The drawing under review shows one solid part. Ordinate dimensions are in mm from its lowest x, y, z. A direction names the side the tool comes from. Coordinates: 2 decimals unless noted, no trailing zeros. Loops run counter-clockwise (first coordinate to the right, second up) from the corner with the lowest first, then second, coordinate; pieces in that order, holes last. Notation, with made-up numbers: (11.25, 32) -> (50.25, 32) arc R21 ccw to (50.25, 61) -> close; hole circle Ø9 at (89, 65.5). An arc over 180 degrees is marked (long way). Use a Markdown table: item, result.
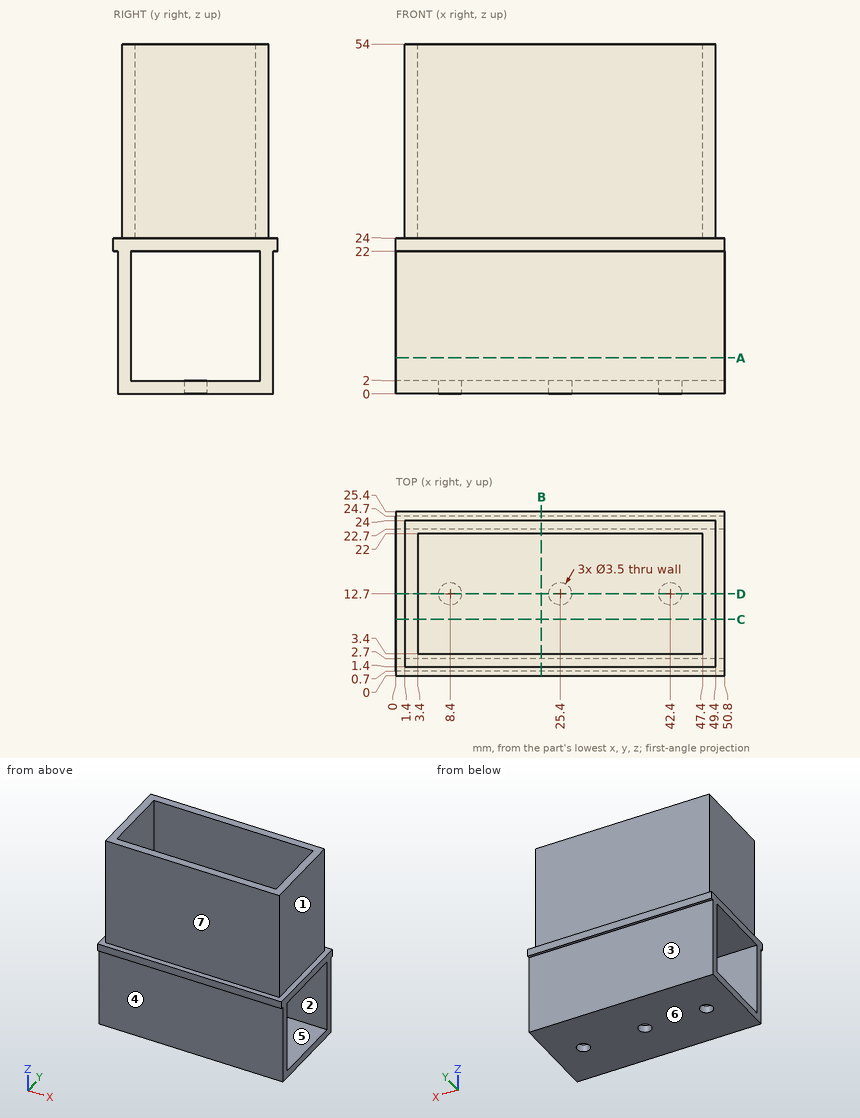
(1) For the marked faces 1, 2, 3 and 4, list the 3-axis set-ups (+Z, -Z, +X, -X, +Y, -Y) from which the entire face can be reached by the end or side of a thin tool; tool diameter is ignored.
Found:
| item | result |
|---|---|
| face 1 | +Z, +X, +Y, -Y |
| face 2 | +X, -X |
| face 3 | -Z, +X, -X, +Y |
| face 4 | -Z, +X, -X, -Y |
(2) Take a section at D-D on y = 12.7. Write out the cut boundary in (x, z), plus the area to 3 significant figures.
Found:
| item | result |
|---|---|
| outline | (0, 0) -> (6.65, 0) -> (6.65, 2) -> (0, 2) -> close; (0, 22) -> (50.8, 22) -> (50.8, 24) -> (49.4, 24) -> (49.4, 54) -> (47.4, 54) -> (47.4, 24) -> (3.4, 24) -> (3.4, 54) -> (1.4, 54) -> (1.4, 24) -> (0, 24) -> close; (10.15, 0) -> (23.65, 0) -> (23.65, 2) -> (10.15, 2) -> close; (27.15, 0) -> (40.65, 0) -> (40.65, 2) -> (27.15, 2) -> close; (44.15, 0) -> (50.8, 0) -> (50.8, 2) -> (44.15, 2) -> close |
| area | 302 mm^2 |
(3) For pin 1 Ø8 at (x, y) = (33.5, 14.5) entering from +Z; pin 2 Ø22 at (x, z) = (32, 7.5) entering from -Y; pin 3 Ø2 at (x, y) = (40, 8) entering from -Z; pin 4 Ø9 at (x, z) = (27, 43.5) entering from +Y, all flat-tipped, find the tip position at first contact; note any pin that passes through.
Found:
| item | result |
|---|---|
| pin 1 | stops at z = 24 |
| pin 2 | stops at y = 0.7 |
| pin 3 | stops at z = 0 |
| pin 4 | stops at y = 24 |
(4) For line 1 along Y through (x, z) = (18.5, 28.5); line 2 along Z through (x, y) = (32.5, 9.5); line 3 along X through (y, z) = (19.25, 31), list the stretches that pass through material, from the lowest coordinate up.
Found:
| item | result |
|---|---|
| line 1 | y = 1.4 to 3.4, 22 to 24 |
| line 2 | z = 0 to 2, 22 to 24 |
| line 3 | x = 1.4 to 3.4, 47.4 to 49.4 |
(5) Take a section at C-C on y = 8.75. Write out the cut boundary in (x, z), plus the area to 3 significant figures.
Found:
| item | result |
|---|---|
| outline | (0, 0) -> (50.8, 0) -> (50.8, 2) -> (0, 2) -> close; (0, 22) -> (50.8, 22) -> (50.8, 24) -> (49.4, 24) -> (49.4, 54) -> (47.4, 54) -> (47.4, 24) -> (3.4, 24) -> (3.4, 54) -> (1.4, 54) -> (1.4, 24) -> (0, 24) -> close |
| area | 323 mm^2 |
(6) Take a section at B-B on x = 22.5. Write out the cut boundary in (y, z), plus the area to 3 significant figures.
Found:
| item | result |
|---|---|
| outline | (0, 22) -> (0.7, 22) -> (0.7, 0) -> (24.7, 0) -> (24.7, 22) -> (25.4, 22) -> (25.4, 24) -> (24, 24) -> (24, 54) -> (22, 54) -> (22, 24) -> (3.4, 24) -> (3.4, 54) -> (1.4, 54) -> (1.4, 24) -> (0, 24) -> close; hole (2.7, 2) -> (22.7, 2) -> (22.7, 22) -> (2.7, 22) -> close |
| area | 299 mm^2 |
(7) Take a section at A-A on z = 5.5. Write out the cut boundary in (x, y).
Found:
| item | result |
|---|---|
| outline | (0, 0.7) -> (50.8, 0.7) -> (50.8, 2.7) -> (0, 2.7) -> close; (0, 22.7) -> (50.8, 22.7) -> (50.8, 24.7) -> (0, 24.7) -> close |
(8) Mouldability with a two-part tool opening along Z and no side actions: class the marked faces 5, 6 and 7 as pulls with the +Z half, pulls with the -Z half, needs draft (parallel to the pull), parting line crosses it, or undercut.
Found:
| item | result |
|---|---|
| face 5 | undercut |
| face 6 | pulls with the -Z half |
| face 7 | needs draft |
